Source: CAD feature listing. Evaluate the final solid. Frame: model axes, mm. A direction names the side the tool comes from. Round coordinates to 2 decimals unless told otherwise and drop trailing zeros. Order: outer loops, then holes, each group sorted by start corner. A loop starts at its lowest first (then second) coordinate and runs counter-clockwise, first axis right, second up. Notation, with made-up numbers: (-12.75, 66.25) - (17.25, 66.25) arc R17 ccw to (17.25, 72.25) - close; hole circle Ø6 at (60, 35). An arc over 180 degrees is marked (long way). Return JSON: item names as keys, results as strings. Group by question number.
1) Section A-A, the plane x = 28. Return loops of the section in (y, z), plus the area to 3 significant figures.
2) Section C-C, the plane y = 0. Return loops of the section in (x, z), plus the area to 3 significant figures.
3) Access query for faces 1 (the flat face through (47, -22, 29)), 2 (the flat face through (-49, -4, 4)), 3 (the flat face through (-11, -29, 0)). Directions: +Z, -Z, +X, -X, +Y, -Y. A direction counts if a zero-diameter tool reaches every point of the face in a straight line with its end or side. Return the directions, or none.
4) Ray query, line 1 (Y direction, x = -45, z = 35); line 2 (X direction, y = 25, z = 32); line 3 (X direction, y = 7, z = 40). Return the intervals inside material, ascending. Write a range as from..to.
5) Section D-D, the plane x = -13.5. Return loops of the section in (y, z), plus the area to 3 significant figures.
6) Mould query, pull axis X, two halves, no side actions, for faces 4 (the flat face through (-50, 0, 30)), 5 (the flat face through (45, 25, 58)), 6 (the flat face through (-1, -30, 30)). Classes: pulls with the +X half, pulls with the -X half, needs draft (parallel to the pull), parting line crosses it, or undercut.
7) Section B-B, the plane z = 21.5. Return loops of the section in (x, y), plus the area to 3 significant figures.
8) Contact query for flat-ended pins moving along their axis: P1, Ø4.5, axis at x = -24, y = 0, coming from the +Z side; P2, Ø2.5, axis at x = 45, y = 25, coming from the -Z side. Output: stop coordinate, or through.
```python
from build123d import *

# Parameters (mm, degrees)
SKETCH1_W               = 100
SKETCH1_H               = 60
BOSS_EXTRUDE1_DEPTH     = 60
SHELL1_T                = -2
SKETCH2_R               = 3.75
SKETCH2_R_2             = 4
CUT_EXTRUDE1_DEPTH      = 60
SKETCH3_R               = 1.35
BOSS_EXTRUDE4_DEPTH     = 58
MIRROR2_COPY_1_SKETCH_R = 1.35
MIRROR2_COPY_1_DEPTH    = 58
FILLET1_R               = 1
CUT_EXTRUDE2_DEPTH      = 121.415945788


with BuildPart() as part:
    # Sketch1 → Boss-Extrude1 (new body)
    with BuildSketch(Plane.XY):
        Rectangle(SKETCH1_W, SKETCH1_H)
    extrude(amount=BOSS_EXTRUDE1_DEPTH)

    # Shell1
    shell1_openings = [part.faces().sort_by_distance(p)[0] for p in [
        (0, 0, 0),
    ]]
    offset(amount=SHELL1_T, openings=shell1_openings, kind=Kind.INTERSECTION)

    # Sketch2 → Cut-Extrude1 (cut)
    with BuildSketch(Plane.XY.offset(60)):
        with Locations((-24, 0)):
            Circle(SKETCH2_R)
        with Locations((28, 0)):
            Circle(SKETCH2_R_2)
    extrude(amount=-CUT_EXTRUDE1_DEPTH, mode=Mode.SUBTRACT)

    # Sketch3 → Boss-Extrude4 (add)
    with BuildSketch(Plane(origin=(0, 0, 58), x_dir=(-1, 0, 0), z_dir=(0, 0, -1))):
        with BuildLine():
            Line((-42, 25), (-42, 28))
            Line((-42, 28), (-48, 28))
            Line((-48, 28), (-48, 22))
            Line((-48, 22), (-45, 22))
            ThreePointArc((-45, 22), (-42.878679656, 22.878679656), (-42, 25))
        make_face()
        with Locations(Location((-45, 25, 0), (0, 0, 180))):
            Circle(SKETCH3_R, mode=Mode.SUBTRACT)
    boss_extrude4 = extrude(amount=BOSS_EXTRUDE4_DEPTH)

    # Mirror1: Boss-Extrude4 across plane
    add(boss_extrude4.mirror(Plane(origin=(0, 0, 0), x_dir=(0, 0, 1), z_dir=(1, 0, 0))))

    # Mirror2: Boss-Extrude4 across plane
    add(boss_extrude4.mirror(Plane.ZX))

    # Mirror2 copy 1 sketch → Mirror2 copy 1 (add)
    with BuildSketch(Plane(origin=(0, 0, 58), x_dir=(1, 0, 0), z_dir=(0, 0, -1))):
        with BuildLine():
            Line((-42, 25), (-42, 28))
            Line((-42, 28), (-48, 28))
            Line((-48, 28), (-48, 22))
            Line((-48, 22), (-45, 22))
            ThreePointArc((-45, 22), (-42.878679656, 22.878679656), (-42, 25))
        make_face()
        with Locations(Location((-45, 25, 0), (0, 0, 180))):
            Circle(MIRROR2_COPY_1_SKETCH_R, mode=Mode.SUBTRACT)
    extrude(amount=MIRROR2_COPY_1_DEPTH)

    # Fillet1
    fillet1_edges = [part.edges().sort_by_distance(p)[0] for p in [
        (-50, 30, 30),
        (50, 30, 30),
        (50, -30, 30),
        (-50, -30, 30),
    ]]
    fillet(fillet1_edges, radius=FILLET1_R)

    # Sketch4 → Cut-Extrude2 (cut, through all)
    with BuildSketch(Plane(origin=(50, 0, 0), x_dir=(0, 0, -1), z_dir=(1, 0, 0))):
        with BuildLine():
            Line((-8, -4), (0, -4))
            Line((0, -4), (0, 4))
            Line((0, 4), (-8, 4))
            ThreePointArc((-8, 4), (-12, 0), (-8, -4))
        make_face()
    extrude(amount=-CUT_EXTRUDE2_DEPTH, mode=Mode.SUBTRACT)


solid = part.part
```
Geometry check:
{
 "1": {"outline": "(-30, 0) - (-28, 0) - (-28, 58) - (-4, 58) - (-4, 60) - (-30, 60) - close; (4, 58) - (28, 58) - (28, 0) - (30, 0) - (30, 60) - (4, 60) - close", "area": "336 mm2"},
 "2": {"outline": "(-50, 12) - (-48, 12) - (-48, 58) - (-27.75, 58) - (-27.75, 60) - (-50, 60) - close; (-20.25, 58) - (24, 58) - (24, 60) - (-20.25, 60) - close; (32, 58) - (48, 58) - (48, 12) - (50, 12) - (50, 60) - (32, 60) - close", "area": "353 mm2"},
 "3": {"face 1": "-Z", "face 2": "-Z, +X, -X", "face 3": "-Z, +X, -X, +Y, -Y"},
 "4": {"line 1": "-30..-26.35, -23.65..-22, 22..23.65, 26.35..30", "line 2": "-50..-46.35, -43.65..-42, 42..43.65, 46.35..50", "line 3": "-50..-48, 48..50"},
 "5": {"outline": "(-30, 0) - (-28, 0) - (-28, 58) - (28, 58) - (28, 0) - (30, 0) - (30, 60) - (-30, 60) - close", "area": "352 mm2"},
 "6": {"face 4": "pulls with the -X half", "face 5": "undercut", "face 6": "needs draft"},
 "7": {"outline": "(-50, -29) arc R1 ccw to (-49, -30) - (49, -30) arc R1 ccw to (50, -29) - (50, 29) arc R1 ccw to (49, 30) - (-49, 30) arc R1 ccw to (-50, 29) - close; hole (-48, -22) - (-45, -22) arc R3 cw to (-42, -25) - (-42, -28) - (42, -28) - (42, -25) arc R3 cw to (45, -22) - (48, -22) - (48, 22) - (45, 22) arc R3 cw to (42, 25) - (42, 28) - (-42, 28) - (-42, 25) arc R3 cw to (-45, 22) - (-48, 22) - close; hole circle Ø2.7 at (-45, -25); hole circle Ø2.7 at (-45, 25); hole circle Ø2.7 at (45, -25); hole circle Ø2.7 at (45, 25)", "area": "737 mm2"},
 "8": {"P1": "through", "P2": "z = 58"}
}
